Geometry check sheet. Reference: the model listing, model coordinates, mm. A direction names the side the tool comes from. Give positions to 0.01 mm unless a question says otherwise; leave off trailing zeros. Loops run counter-clockwise (first coordinate to the right, second up) from the corner with the lowest first, then second, coordinate; pieces in that order, holes last.
```python
from build123d import *

# Parameters (mm, degrees)
F0_W     = 66.04
F0_H     = 218.44
F0_W_2   = 63.5
F0_H_2   = 215.9
F1_DEPTH = 1.27
F2_DEPTH = 50.8
F4_DEPTH = 76.2


with BuildPart() as f1:
    # F0 (on Top) → F1 (new body)
    with BuildSketch(Plane.XY):
        Rectangle(F0_W, F0_H)
        Rectangle(F0_W_2, F0_H_2, mode=Mode.SUBTRACT)
        Rectangle(F0_W_2, F0_H_2)
    extrude(amount=F1_DEPTH)

    # F0 (on Top) → F2 (join)
    with BuildSketch(Plane.XY):
        Rectangle(F0_W, F0_H)
        Rectangle(F0_W_2, F0_H_2, mode=Mode.SUBTRACT)
    extrude(amount=F2_DEPTH)

    # F3 (on face) → F4 (cut)
    with BuildSketch(Plane(origin=(-33.02, 0, 0), x_dir=(0, -1, 0), z_dir=(-1, 0, 0))):
        Polygon((-80.645, 6.35), (-99.695, 44.45), (-99.695, 6.35), align=None)
        Polygon((-74.295, 6.35), (-55.245, 6.35), (-74.295, 44.45), align=None)
        Polygon((-48.895, 6.35), (-29.845, 6.35), (-48.895, 44.45), align=None)
        Polygon((-23.495, 6.35), (-4.445, 6.35), (-23.495, 44.45), align=None)
        Polygon((1.905, 6.35), (20.955, 6.35), (1.905, 44.45), align=None)
        Polygon((27.305, 6.35), (46.355, 6.35), (27.305, 44.45), align=None)
        Polygon((52.705, 6.35), (71.755, 6.35), (52.705, 44.45), align=None)
        Polygon((78.105, 6.35), (97.155, 6.35), (78.105, 44.45), align=None)
    extrude(amount=-F4_DEPTH, mode=Mode.SUBTRACT)


solid = f1.part
```
1) Tool access check on faces 4 (the flat face through (0, 107.95, 26)), 5 (the flat face through (33.02, -26, 25)), 6 (the flat face through (-32.394, -11.563, 25.133)). Record the directions out of +Z, -Z, +X, -X, +Y, -Y that give a thin tool (end or side, any length) a straight path to the whole face; none if there is none.
2) Sectioned sample at A-A on y = 41. Enter the section's corners in (x, z), plus the area to 3 significant figures.
3) Sectioned sample at C-C on y = -69. Enter the section's corners in (x, z).
4) Scan lines: line 1 along Y through (x, z) = (-26, 3.5); line 2 along X through (y, z) = (-16, 4.5); line 3 along Z through (x, y) = (-26.5, -33). Record each from-to range of solid material in increasing order.
5) Sectioned sample at B-B on z = 22. Count the separate pieces of the cut face and the enclosed holes in it, plus the area to 3 significant figures.
6) Mould release check, pull along Y, two halves, no side actions. Record for faces 1 (the flat face through (-33.02, -26, 25)), 2 (the flat face through (32.376, -87.763, 25.133)), 3 (the flat face through (0, -109.22, 25)): +Y half, -Y half, draft (parallel to the pull), parting line (faces both ways), or undercut.
7) Sectioned sample at D-D on x = 25.5. Enter the section's corners in (y, z), plus the area to 3 significant figures.
8) Depth check by flat-ended pin: P1, Ø1, axis at x = -8.5, y = -42, coming from the +Z side. Enter the tip coordinate at first touch or a pass-through.
Determined:
1. face 4: +Z
1. face 5: +Z, -Z, +X, +Y, -Y
1. face 6: +X, -X
2. outline: (-33.02, 0) - (33.02, 0) - (33.02, 6.35) - (31.75, 6.35) - (31.75, 1.27) - (-31.75, 1.27) - (-31.75, 6.35) - (-33.02, 6.35) - close; (-33.02, 28.66) - (-31.75, 28.66) - (-31.75, 50.8) - (-33.02, 50.8) - close; (31.75, 28.66) - (33.02, 28.66) - (33.02, 50.8) - (31.75, 50.8) - close
2. area: 153 mm2
3. outline: (-33.02, 0) - (33.02, 0) - (33.02, 6.35) - (31.75, 6.35) - (31.75, 1.27) - (-31.75, 1.27) - (-31.75, 6.35) - (-33.02, 6.35) - close; (-33.02, 11.86) - (-31.75, 11.86) - (-31.75, 50.8) - (-33.02, 50.8) - close; (31.75, 11.86) - (33.02, 11.86) - (33.02, 50.8) - (31.75, 50.8) - close
4. line 1: y = -109.22 to -107.95, 107.95 to 109.22
4. line 2: x = -33.02 to -31.75, 31.75 to 33.02
4. line 3: z = 0 to 1.27
5. separate pieces: 16
5. enclosed holes: 0
5. area: 488 mm2
6. face 1: draft
6. face 2: undercut
6. face 3: -Y half
7. outline: (-109.22, 0) - (109.22, 0) - (109.22, 50.8) - (107.95, 50.8) - (107.95, 1.27) - (-107.95, 1.27) - (-107.95, 50.8) - (-109.22, 50.8) - close
7. area: 403 mm2
8. P1: stops at z = 1.27
